Autodesk Inventor part; units mm, degrees
ref_plane "YZ Plane" through (0, 0, 0) normal (1, 0, 0) x (0, 1, 0)
ref_plane "XZ Plane" through (0, 0, 0) normal (0, 1, 0) x (-1, 0, 0)
ref_plane "XY Plane" through (0, 0, 0) normal (0, 0, 1) x (1, 0, 0)
sketch "Sketch1" plane through (0, 0, 0) normal (0, 1, 0) x (-1, 0, 0)
  line L0 (0, 0) -> (69, 0)
  line L1 (69, 0) -> (69, -15)
  line L2 (69, -15) -> (0, -15)
  line L3 (0, -15) -> (0, 0)
  dimension "d0" = 69
  dimension "d1" = 15
extrude "Extrusion1" add sketch "Sketch1" along normal blind 3.18
sketch "Sketch2" plane through (0, 0, 0) normal (0, 1, 0) x (-1, 0, 0)
  line L0 (69, 0) -> (0, 0)
  line L1 (0, 0) -> (0, -15)
  line L2 (0, -15) -> (69, -15)
  line L3 (69, -15) -> (69, 0)
  line L4 (0, -15) -> (72.18, -15)
  line L5 (72.18, -15) -> (72.18, -18.18)
  line L6 (72.18, -18.18) -> (0, -18.18)
  line L7 (0, -18.18) -> (0, -15)
  line L8 (72.18, -15) -> (69, -15)
  line L9 (69, -15) -> (69, 0)
  line L10 (69, 0) -> (72.18, 0)
  line L11 (72.18, 0) -> (72.18, -15)
  line L12 (0, 0) -> (20, 0)
  line L13 (20, 0) -> (20, 3.18)
  line L14 (20, 3.18) -> (0, 3.18)
  line L15 (0, 3.18) -> (0, 0)
  line L16 (20, 0) -> (50, 0)
  line L17 (50, 0) -> (50, 3.18)
  line L18 (20, 3.18) -> (20, 0)
  line L19 (50, 3.18) -> (72.18, 3.18)
  line L20 (72.18, 3.18) -> (72.18, 0)
  line L21 (72.18, 0) -> (50, 0)
  line L22 (50, 0) -> (50, 3.18)
  dimension "d4" = 72.18
  dimension "d5" = 3.18
  dimension "d6" = 20
  dimension "d7" = 3.18
  dimension "d9" = 22.18
extrude "Extrusion2" add sketch "Sketch2" along normal blind 56.18 contours L10 L11 L4 L3 | L0 L17 L19 L20 L10 | L4 L5 L6 L7 L2 | L0 L15 L14 L13
sketch "Sketch3" plane through (0, 56.18, 0) normal (0, 1, 0) x (1, 0, 0)
  line L0 (0, 0) -> (-20, 0)
  line L1 (-20, 0) -> (-20, -3.18)
  line L2 (-20, -3.18) -> (0, -3.18)
  line L3 (0, -3.18) -> (0, 0)
  line L4 (-69, 0) -> (-69, 15)
  line L5 (-69, 15) -> (0, 15)
  line L6 (0, 15) -> (0, 18.18)
  line L7 (0, 18.18) -> (-72.18, 18.18)
  line L8 (-72.18, 18.18) -> (-72.18, -3.18)
  line L9 (-72.18, -3.18) -> (-50, -3.18)
  line L10 (-50, -3.18) -> (-50, 0)
  line L11 (-50, 0) -> (-69, 0)
  line L12 (0, -3.18) -> (-72.18, -3.18)
  line L13 (-72.18, -3.18) -> (-72.18, 18.18)
  line L14 (-72.18, 18.18) -> (0, 18.18)
  line L15 (0, 18.18) -> (0, -3.18)
extrude "Extrusion3" add sketch "Sketch3" along normal blind 3.18
properties part number "Base_Arduino"
Could you check a few things on this model? Use its own coordinates, in mm. A direction names the side the tool comes from. Round coordinates to 2 decimals unless told otherwise and drop trailing zeros. Write each loop counter-clockwise with the first axis right and the second up, starting at its lowest first coordinate (ties: lowest second). Pieces come first, ordered by that corner, then holes. Notation, with made-up numbers: (-39.75, 64.25) -> (-6.75, 64.25) arc R15 cw to (-6.75, 92.25) -> close; hole circle Ø3 at (34, 85.5). An arc over 180 degrees is marked (long way). Use a Markdown table: item, result.
1. If we section it at C-C (z = -2.5): List the corners of the cut face in (x, y) for me, then the cut area to 3 significant figures.
Answer key:
| item | result |
|---|---|
| outline | (-72.18, 0) -> (0, 0) -> (0, 3.18) -> (-69, 3.18) -> (-69, 56.18) -> (0, 56.18) -> (0, 59.36) -> (-72.18, 59.36) -> close |
| area | 628 mm^2 |
2. For pin 1 Ø16 at (x, y) = (-36.5, 32.5) entering from +Z; pin 2 Ø1 at (x, y) = (-35.5, 1) entering from +Z, each with a flat end and sliding along its axis, tell me the tip position at first contact or that it passes through.
Answer key:
| item | result |
|---|---|
| pin 1 | stops at z = -15 |
| pin 2 | stops at z = 0 |
3. Please list where these lines run through material, in increasing order: probe 1 along Z at (x, y) = (-59, 10.5); probe 2 along Y at (x, z) = (-56, -9.25); probe 3 along X at (y, z) = (35, -6.75).
Answer key:
| item | result |
|---|---|
| probe 1 | z = -18.18 to -15, 0 to 3.18 |
| probe 2 | y = 0 to 3.18, 56.18 to 59.36 |
| probe 3 | x = -72.18 to -69 |
4. Which directions (+Z, -Z, +X, -X, +Y, -Y) give clear straight access to the entire face, cutting with the end or side of a thin tool? Please do faces 5 (the face through (-35, 2, 0)), 6 (the face through (-34, 29, -15)), 7 (the face through (0, 25.1, 0.4)).
Answer key:
| item | result |
|---|---|
| face 5 | +Z, -Y |
| face 6 | +X |
| face 7 | +Z, -Z, +X, +Y, -Y |
5. If we section it at D-D (x = -37): List the corners of the cut face in (y, z) for me.
Answer key:
| item | result |
|---|---|
| outline | (0, -18.18) -> (59.36, -18.18) -> (59.36, 3.18) -> (56.18, 3.18) -> (56.18, -15) -> (3.18, -15) -> (3.18, 0) -> (0, 0) -> close |
6. We'd pull the mould along Y, two halves only. Please class faces 1 (the face through (-34, 3.18, -7)), 2 (the face through (-36, 0, -7)), 3 (the face through (-50, 28, 2)), 4 (the face through (-37, 59.36, -8)): +Y half, -Y half, draft (parallel to the pull), parting line (faces both ways), or undercut.
Answer key:
| item | result |
|---|---|
| face 1 | undercut |
| face 2 | -Y half |
| face 3 | draft |
| face 4 | +Y half |
7. If we section it at A-A (y = 50.5): List the corners of the cut face in (x, z) for me, then the cut area to 3 significant figures.
Answer key:
| item | result |
|---|---|
| outline | (-72.18, -18.18) -> (0, -18.18) -> (0, -15) -> (-69, -15) -> (-69, 0) -> (-50, 0) -> (-50, 3.18) -> (-72.18, 3.18) -> close; (-20, 0) -> (0, 0) -> (0, 3.18) -> (-20, 3.18) -> close |
| area | 411 mm^2 |
8. If we section it at B-B (x = -62.5): List the corners of the cut face in (y, z) for me, then the cut area to 3 significant figures.
Answer key:
| item | result |
|---|---|
| outline | (0, -18.18) -> (59.36, -18.18) -> (59.36, 3.18) -> (0, 3.18) -> close; hole (3.18, -15) -> (56.18, -15) -> (56.18, 0) -> (3.18, 0) -> close |
| area | 473 mm^2 |
